Geometry check sheet. Reference: the model listing, model coordinates, mm. Round coordinates to 2 decimals unless told otherwise and drop trailing zeros. Loops run counter-clockwise (first coordinate to the right, second up) from the corner with the lowest first, then second, coordinate; pieces in that order, holes last. Notation, with made-up numbers: (42, 67) - (73, 67) arc R11 cw to (73, 75) - close; hole circle Ø6 at (-12.75, 35). An arc over 180 degrees is marked (long way). Answer as CSV lines item,"result". Start each with the question number.
1) Depth check by flat-ended pin: P1, Ø0.5, axis at x = 28.5, z = 0.5, coming from the +Y side; P2, Ø0.5, axis at y = 27, z = 0.5, coming from the +X side; P3, Ø0.5, axis at y = 23.5, z = 0.5, coming from the -X side. Enter the tip coordinate at first touch or a pass-through.
2) Cross-section at B-B on x = 0. Record the boundary of the cut face in (y, z), and give its area (3 significant figures).
3) Cross-section at A-A on z = 0.3. State how many separate pieces and enclosed holes the cut face has, and give its area (3 significant figures).
4) Cross-section at D-D on x = 31. Record the boundary of the cut face in (y, z), and give its area (3 significant figures).
5) Thickness scan on line 1 along Y through (x, z) = (27.5, 0.65); line 2 along X through (y, z) = (-9, 0.95); line 3 along Y through (x, z) = (10.5, 0.35). Record the ranges inside material, lowest first.
from build123d import *

# Parameters (mm, degrees)
SKETCH1_R           = 2
SKETCH1_W           = 56
SKETCH1_H           = 56
BOSS_EXTRUDE1_DEPTH = 1
CHAMFER1_SIZE       = 2


with BuildPart() as part:
    # Sketch1 → Boss-Extrude1 (new body)
    with BuildSketch(Plane.XY):
        with BuildLine():
            Line((40, -13), (40, 13))
            ThreePointArc((40, 13), (38.828427125, 15.828427125), (36, 17))
            ThreePointArc((36, 17), (33.171572875, 18.171572875), (32, 21))
            Line((32, 21), (32, 32))
            Line((32, 32), (21, 32))
            ThreePointArc((21, 32), (18.171572875, 33.171572875), (17, 36))
            ThreePointArc((17, 36), (15.828427125, 38.828427125), (13, 40))
            Line((13, 40), (-13, 40))
            ThreePointArc((-13, 40), (-15.828427125, 38.828427125), (-17, 36))
            ThreePointArc((-17, 36), (-18.171572875, 33.171572875), (-21, 32))
            Line((-21, 32), (-32, 32))
            Line((-32, 32), (-32, 9))
            ThreePointArc((-32, 9), (-33.464466094, 5.464466094), (-37, 4))
            ThreePointArc((-37, 4), (-41, 0), (-37, -4))
            ThreePointArc((-37, -4), (-33.464466094, -5.464466094), (-32, -9))
            Line((-32, -9), (-32, -32))
            Line((-32, -32), (-9, -32))
            ThreePointArc((-9, -32), (-5.464466094, -33.464466094), (-4, -37))
            ThreePointArc((-4, -37), (0, -41), (4, -37))
            ThreePointArc((4, -37), (5.464466094, -33.464466094), (9, -32))
            Line((9, -32), (32, -32))
            Line((32, -32), (32, -21))
            ThreePointArc((32, -21), (33.171572875, -18.171572875), (36, -17))
            ThreePointArc((36, -17), (38.828427125, -15.828427125), (40, -13))
        make_face()
        with Locations((-37, 0)):
            Circle(SKETCH1_R, mode=Mode.SUBTRACT)
        with Locations((-13, 36)):
            Circle(SKETCH1_R, mode=Mode.SUBTRACT)
        with Locations((0, -37)):
            Circle(SKETCH1_R, mode=Mode.SUBTRACT)
        with Locations((36, -13)):
            Circle(SKETCH1_R, mode=Mode.SUBTRACT)
        with Locations((36, 13)):
            Circle(SKETCH1_R, mode=Mode.SUBTRACT)
        with Locations((13, 36)):
            Circle(SKETCH1_R, mode=Mode.SUBTRACT)
        Rectangle(SKETCH1_W, SKETCH1_H, mode=Mode.SUBTRACT)
    extrude(amount=BOSS_EXTRUDE1_DEPTH)

    # Chamfer1
    # the kernel refuses this chamfer: 2 mm, written as the material it takes off along each edge
    with BuildSketch(Plane(origin=(13, 36, 1), x_dir=(1, 0, 0), z_dir=(0, -1, 0))) as chamfer1_piece_1:
        Polygon((2, -CHAMFER1_SIZE), (2 + CHAMFER1_SIZE, 0), (2, 0), align=None)
    revolve(axis=Axis((13, 36, 1), (0, 0, 1)), mode=Mode.SUBTRACT)
    with BuildSketch(Plane(origin=(-13, 36, 1), x_dir=(1, 0, 0), z_dir=(0, -1, 0))) as chamfer1_piece_2:
        Polygon((2, -CHAMFER1_SIZE), (2 + CHAMFER1_SIZE, 0), (2, 0), align=None)
    revolve(axis=Axis((-13, 36, 1), (0, 0, 1)), mode=Mode.SUBTRACT)
    with BuildSketch(Plane(origin=(-37, 0, 1), x_dir=(1, 0, 0), z_dir=(0, -1, 0))) as chamfer1_piece_3:
        Polygon((2, -CHAMFER1_SIZE), (2 + CHAMFER1_SIZE, 0), (2, 0), align=None)
    revolve(axis=Axis((-37, 0, 1), (0, 0, 1)), mode=Mode.SUBTRACT)
    with BuildSketch(Plane(origin=(36, -13, 1), x_dir=(1, 0, 0), z_dir=(0, -1, 0))) as chamfer1_piece_4:
        Polygon((2, -CHAMFER1_SIZE), (2 + CHAMFER1_SIZE, 0), (2, 0), align=None)
    revolve(axis=Axis((36, -13, 1), (0, 0, 1)), mode=Mode.SUBTRACT)
    with BuildSketch(Plane(origin=(0, -37, 1), x_dir=(1, 0, 0), z_dir=(0, -1, 0))) as chamfer1_piece_5:
        Polygon((2, -CHAMFER1_SIZE), (2 + CHAMFER1_SIZE, 0), (2, 0), align=None)
    revolve(axis=Axis((0, -37, 1), (0, 0, 1)), mode=Mode.SUBTRACT)
    with BuildSketch(Plane(origin=(36, 13, 1), x_dir=(1, 0, 0), z_dir=(0, -1, 0))) as chamfer1_piece_6:
        Polygon((2, -CHAMFER1_SIZE), (2 + CHAMFER1_SIZE, 0), (2, 0), align=None)
    revolve(axis=Axis((36, 13, 1), (0, 0, 1)), mode=Mode.SUBTRACT)


solid = part.part
Answer block:
1,P1,"stops at y = 32"
1,P2,"stops at x = 32"
1,P3,"stops at x = -32"
2,outline,"(-41, 0) - (-40, 0) - (-41, 1) - close; (-34, 0) - (-28, 0) - (-28, 1) - (-33, 1) - close; (28, 0) - (40, 0) - (40, 1) - (28, 1) - close"
2,area,"18.0 mm^2"
3,separate pieces,"1"
3,enclosed holes,"7"
3,area,"1,450 mm^2"
4,outline,"(-32, 0) - (32, 0) - (32, 1) - (-32, 1) - close"
4,area,"64.0 mm^2"
5,line 1,"y = -32 to -28, 28 to 32"
5,line 2,"x = -32 to -28, 28 to 40"
5,line 3,"y = -32 to -28, 28 to 33.77, 38.23 to 40"
